Work out the finished part from the listing and answer in its coordinate system (mm). A direction names the side the tool comes from. Coordinates: 2 decimals unless noted, no trailing zeros. Order: outer loops, then holes, each group sorted by start corner. A loop starts at its lowest first (then second) coordinate and runs counter-clockwise, first axis right, second up. Notation, with made-up numbers: (-23.5, 48.5) - (-12.5, 48.5) arc R18 cw to (-12.5, 77.5) - close; hole circle Ø4 at (75, -33). An arc over 180 degrees is marked (long way). Answer as a JSON object with one key per item and string values. Group by question number.
1) Section C-C (x = -9.5) is taken. Give the vertices of the cut face in (y, z), plus the area to 3 significant figures.
2) Each of these flat-tipped pins is pushed along its axis until it touches: P1, Ø3.5, axis at y = -15.5, z = 24, coming from the -X side; P2, Ø1, axis at x = 6, z = 26.5, coming from the -Y side; P3, Ø8, axis at x = 3, z = 18, coming from the -Y side; P4, Ø1.5, axis at x = 5.5, y = 11.5, coming from the -Z side. Where does it stop, or does it pass through?
3) A tool of negligible diameter and unlimited length cuts with its end or side. For faces 1 (the face through (0, -17.788, 27)), 2 (the face through (0, -18.223, 20)), 3 (the face through (2.5, -18, 24)), from which of +Z, -Z, +X, -X, +Y, -Y can it reach the whole face along a straight path? Write none if from no direction.
4) Section D-D (z = 12.5) is taken. Give the vertices of the cut face in (x, y), plus the area to 3 significant figures.
5) Section B-B (y = 5) is taken. Give the vertices of the cut face in (x, z).
6) The mould has two halves that part along Z. Classify faces 4 (the face through (0, -16, 16.289)), 5 (the face through (0, -19.225, 28)), 6 (the face through (-14, 7, 40)), 7 (the face through (0, -17.05, 20)): released by +Z, released by -Z, zero draft, split by the parting line, or undercut.
7) Section A-A (x = 0) is taken. Give the vertices of the cut face in (y, z).
8) Find the intervals of material crossed by line 1 along Y through (x, z) = (0, 18.5); line 2 along Y through (x, z) = (0, 12); line 3 along X through (y, z) = (10, 25.5), in increasing order.
from build123d import *

# Parameters (mm, degrees)
F0_R     = 18.433835
F0_R_2   = 15.332756
F1_DEPTH = 40
F2_W     = 9.342166
F2_H     = 15.280273
F3_DEPTH = 25
F6_DEPTH = 2.5


with BuildPart() as f1:
    # F0 (on Top) → F1 (new body)
    with BuildSketch(Plane.XY):
        Circle(F0_R)
        Circle(F0_R_2, mode=Mode.SUBTRACT)
    extrude(amount=F1_DEPTH)


with BuildPart() as f3:
    # F2 (on Front) → F3 (new body)
    with BuildSketch(Plane.XZ):
        with Locations((0, 23.92951)):
            Rectangle(F2_W, F2_H)
    extrude(amount=F3_DEPTH)


with BuildPart() as f1_1:
    add(f1.part)

    # F4: cut F3
    add(f3.part, mode=Mode.SUBTRACT)

    # F5 (on Right) → F6 (join, symmetric)
    with BuildSketch(Plane.YZ):
        Polygon((-18.222677, 16.054166), (-18.222677, 0), (-17.050333, 0), (-17.050333, 23.467397), (-17.787579, 26.047755), (-17.787579, 28.786093), (-16.260428, 29.418018), (-16.719699, 30.708198), (-19.224662, 29.580966), (-19.224662, 26.074016), (-18.222677, 23.068061), align=None)
    extrude(amount=F6_DEPTH, both=True)


solid = f1_1.part
Report:
{
 "1": {"outline": "(-15.8, 0) - (-12.04, 0) - (-12.04, 40) - (-15.8, 40) - close; (12.04, 0) - (15.8, 0) - (15.8, 40) - (12.04, 40) - close", "area": "301 mm²"},
 "2": {"P1": "stops at x = -12.28", "P2": "stops at y = -17.59", "P3": "stops at y = -18.43", "P4": "passes through"},
 "3": {"face 1": "none", "face 2": "+X, -X, -Y", "face 3": "-Y"},
 "4": {"outline": "circle Ø36.87 at (0, 0); hole circle Ø30.67 at (0, 0)", "area": "329 mm²"},
 "5": {"outline": "(-17.74, 0) - (-14.49, 0) - (-14.49, 40) - (-17.74, 40) - close; (14.49, 0) - (17.74, 0) - (17.74, 40) - (14.49, 40) - close"},
 "6": {"face 4": "undercut", "face 5": "zero draft", "face 6": "released by +Z", "face 7": "undercut"},
 "7": {"outline": "(-19.22, 26.07) - (-18.22, 23.07) - (-18.22, 16.29) - (-18.43, 16.29) - (-18.43, 0) - (-15.33, 0) - (-15.33, 16.29) - (-17.05, 16.29) - (-17.05, 23.47) - (-17.79, 26.05) - (-17.79, 28.79) - (-16.26, 29.42) - (-16.72, 30.71) - (-19.22, 29.58) - close; (-18.43, 31.57) - (-15.33, 31.57) - (-15.33, 40) - (-18.43, 40) - close; (15.33, 0) - (18.43, 0) - (18.43, 40) - (15.33, 40) - close"},
 "8": {"line 1": "y = -18.22 to -17.05, 15.33 to 18.43", "line 2": "y = -18.43 to -15.33, 15.33 to 18.43", "line 3": "x = -15.49 to -11.62, 11.62 to 15.49"}
}
